```python
from build123d import *

# Parameters (mm, degrees)
F0_W          = 120
F0_H          = 400
F1_DEPTH      = 25
F2_W          = 120
F2_H          = 25
F3_DEPTH      = 200
F4_R          = 35
F5_DEPTH      = 70
F6_R          = 23.205
F7_DEPTH      = 30
F8_W          = 40
F8_H          = 25
F8_W_2        = 120
F9_DEPTH      = 200
F9_DEPTH_BACK = 25
F10_R         = 65
F11_DEPTH     = 50
F12_R         = 13
F13_DEPTH     = 125
F14_R         = 25
F15_DEPTH     = 105
F16_W         = 350
F16_H         = 220
F17_DEPTH     = 15
F18_W         = 215
F18_H         = 7.5
F18_W_2       = 10
F19_DEPTH     = 155
F20_W         = 180
F20_H         = 130
F20_R         = 13
F21_DEPTH     = 7.5
F22_R         = 5


with BuildPart() as f1:
    # F0 (on Front) → F1 (new body)
    with BuildSketch(Plane.XZ):
        Rectangle(F0_W, F0_H)
    extrude(amount=F1_DEPTH)

    # F2 (on face) → F3 (join)
    with BuildSketch(Plane.XZ.offset(25)):
        with Locations((0, 187.5)):
            Rectangle(F2_W, F2_H)
    extrude(amount=F3_DEPTH)

    # F4 (on face) → F5 (join)
    with BuildSketch(Plane(origin=(0, 0, 175), x_dir=(1, 0, 0), z_dir=(0, 0, -1))):
        with Locations((0, 135)):
            Circle(F4_R)
    extrude(amount=F5_DEPTH)

    # F6 (on face) → F7 (join)
    with BuildSketch(Plane(origin=(0, 0, 105), x_dir=(1, 0, 0), z_dir=(0, 0, -1))):
        with Locations((0, 135)):
            Circle(F6_R)
    extrude(amount=F7_DEPTH)

    # F8 (on face) → F9 (join, two sides)
    with BuildSketch(Plane.XZ.offset(25)) as f9_sk:
        with Locations((-80, -187.5)):
            Rectangle(F8_W, F8_H)
        with Locations((0, -187.5)):
            Rectangle(F8_W_2, F8_H)
        with Locations((80, -187.5)):
            Rectangle(F8_W, F8_H)
    extrude(amount=F9_DEPTH)
    extrude(f9_sk.sketch, amount=-F9_DEPTH_BACK)

    # F10 (on face) → F11 (join)
    with BuildSketch(Plane.XY.offset(-175)):
        with Locations((-23.4574452043, -131.4095705748)):
            Circle(F10_R)
    extrude(amount=F11_DEPTH)

    # F12 (on face) → F13 (join)
    with BuildSketch(Plane.XY.offset(-125)):
        with Locations((0, -135)):
            Circle(F12_R)
    extrude(amount=F13_DEPTH)

    # F14 (on face) → F15 (join)
    with BuildSketch(Plane.XY.offset(-125)):
        with Locations((-54.2105034057, -125.7144563701)):
            Circle(F14_R)
    extrude(amount=F15_DEPTH)

    # F16 (on Top) → F17 (join)
    with BuildSketch(Plane.XY):
        with Locations((0, -135)):
            Rectangle(F16_W, F16_H)
        with BuildLine():
            ThreePointArc((117.5, -202.5), (114.5710678119, -209.5710678119), (107.5, -212.5))
            Line((107.5, -212.5), (-107.5, -212.5))
            ThreePointArc((-107.5, -212.5), (-114.5710678119, -209.5710678119), (-117.5, -202.5))
            Line((-117.5, -202.5), (-117.5, -67.5))
            ThreePointArc((-117.5, -67.5), (-114.5710678119, -60.4289321881), (-107.5, -57.5))
            Line((-107.5, -57.5), (107.5, -57.5))
            ThreePointArc((107.5, -57.5), (114.5710678119, -60.4289321881), (117.5, -67.5))
            Line((117.5, -67.5), (117.5, -202.5))
        make_face(mode=Mode.SUBTRACT)
    extrude(amount=-F17_DEPTH)

    # F18 (on face) → F19 (join)
    with BuildSketch(Plane.XZ.offset(57.5)):
        with Locations((0, -11.25)):
            Rectangle(F18_W, F18_H)
        with Locations((-112.5, -11.25)):
            Rectangle(F18_W_2, F18_H)
        with Locations((112.5, -11.25)):
            Rectangle(F18_W_2, F18_H)
    extrude(amount=F19_DEPTH)

    # F20 (on face) → F21 (cut, through all)
    with BuildSketch(Plane.XY.offset(-7.5)):
        with Locations((0, -135)):
            Rectangle(F20_W, F20_H)
        with Locations((0, -135)):
            Circle(F20_R, mode=Mode.SUBTRACT)
    extrude(amount=-F21_DEPTH, mode=Mode.SUBTRACT)

    # F22
    f22_edges = [f1.edges().sort_by_distance(p)[0] for p in [
        (-90, -70, -11.25),
        (90, -70, -11.25),
        (-90, -200, -11.25),
        (90, -200, -11.25),
    ]]
    fillet(f22_edges, radius=F22_R)


solid = f1.part
```
Work out the finished part from the listing and answer in its coordinate system (mm). A direction names the side the tool comes from. Round coordinates to 2 decimals unless told otherwise and drop trailing zeros. Write each loop counter-clockwise with the first axis right and the second up, starting at its lowest first coordinate (ties: lowest second). Pieces come first, ordered by that corner, then holes.
1) Which of the six approach directions +Z, -Z, +X, -X, +Y, -Y give full straight-line access (tool end or side, diameter ignored) to faces 1 (the face through (100, -111, -188)), 2 (the face through (0, -135, 0)), 3 (the face through (-55, -125, -20)), 4 (the face through (-79.186, -124.615, -73.235)), 5 (the face through (-114.49, -209.65, -3.7))?
2) A cutting plane is placed at B-B on y = -91. Determine the outline of the cut face in (x, z), and give its area (3 significant figures).
3) A cutting plane is placed at A-A on z = 155.5. Determine the outline of the cut face in (x, y), and give its area (3 significant figures).
4) Consider probe 1 along X at (y, z) = (-161, -10); probe 2 along Z at (x, y) = (56.5, -207); probe 3 along Z at (x, y) = (2, -234). Determine where each line is inside the solid, lowest interval first.
5) A cutting plane is placed at C-C on x = -151. Determine the outline of the cut face in (y, z).
6) Determine the mould class of faces 6 (the face through (117, -25, -7)), 7 (the face through (-7.587, -100.832, 140.49)), 8 (the face through (-175, -137, -7)), 9 (the face through (-2, -245, -7)) for opening direction Y: pulls with the +Y half, pulls with the -Y half, needs draft (parallel to the pull), parting line crosses it, or undercut.
7) Flat-ended cylindrical pins translate along their axes: P1, Ø3, axis at x = 28, z = -24, coming from the -Y side; P2, Ø8, axis at y = -93, z = -150, coming from the -X side; P3, Ø12, axis at x = 127.5, z = -4.5, coming from the +Y side. Find the tip coordinate at first contact, or state that the pin passes through.
Entries:
1. face 1: -Z, +X, +Y, -Y
1. face 2: +X, -X, -Y
1. face 3: -X, -Y
1. face 4: none
1. face 5: +Z
2. outline: (-175, -15) - (-90, -15) - (-90, -7.5) - (-117.5, -7.5) - (-117.5, 0) - (-175, 0) - close; (-100, -200) - (100, -200) - (100, -175) - (27.45, -175) - (27.45, -125) - (-74.37, -125) - (-74.37, -175) - (-100, -175) - close; (-60, 175) - (60, 175) - (60, 200) - (-60, 200) - close; (90, -15) - (175, -15) - (175, 0) - (117.5, 0) - (117.5, -7.5) - (90, -7.5) - close
2. area: 15,200 mm2
3. outline: (-60, -25) - (60, -25) - (60, 0) - (-60, 0) - close; circle Ø70 at (0, -135)
3. area: 6,850 mm2
4. probe 1: x = -175 to -90, 90 to 175
4. probe 2: z = -200 to -175, -15 to -7.5, 175 to 200
4. probe 3: z = -15 to 0
5. outline: (-245, -15) - (-25, -15) - (-25, 0) - (-245, 0) - close
6. face 6: pulls with the +Y half
6. face 7: undercut
6. face 8: needs draft
6. face 9: pulls with the -Y half
7. P1: stops at y = -25
7. P2: stops at x = -78.6
7. P3: stops at y = -25
